from build123d import *

# Parameters (mm, degrees)
F0_R     = 114.3
F1_DEPTH = 15.24
F3_D     = 76.2
F5_D     = 20.32
F7_D     = 20.32


with BuildPart() as f1:
    # F0 (on Front) → F1 (new body)
    with BuildSketch(Plane.XZ):
        Circle(F0_R)
    extrude(amount=F1_DEPTH)

    # F3 (through all)
    with Locations(Plane.XZ.offset(15.24)):
        with Locations((0, 0)):
            Hole(F3_D / 2)

    # F5 (through all)
    with Locations(Plane.XZ.offset(15.24)):
        with Locations((0, 76.2)):
            Hole(F5_D / 2)

    # F7 (through all)
    with Locations(Plane.XZ.offset(15.24)):
        with Locations((0, -76.2)):
            Hole(F7_D / 2)


solid = f1.part
Could you check a few things on this model? Use its own coordinates, in mm. Give positions to 0.01 mm unless a question says otherwise; leave off trailing zeros. Order: outer loops, then holes, each group sorted by start corner. A loop starts at its lowest first (then second) coordinate and runs counter-clockwise, first axis right, second up. Notation, with made-up numbers: (57, 27) - (63, 27) arc R18 cw to (63, 31) - close; hole circle Ø4 at (-28.5, 88.5). An arc over 180 degrees is marked (long way). One line per question, with ' | ' between items. Start each with the question number.
Item 1: Thinking about a two-plate mould opening in Z: for faces 1 (the flat face through (-2, 0, -49)), 2 (the cylindrical face through (30.235, -7.513, -23.183)), 3 (the cylindrical face through (-114.19, -7.51, 5.03)), which applies, pulls with the +Z half, pulls with the -Z half, needs draft (parallel to the pull), parting line crosses it, or undercut?
Item 2: I want a section at D-D on y = -7.25. Write out the boundary of the cut face in (x, z).
Item 3: I'm going to push flat-ended pins straight in: pin 1 Ø4 at (y, z) = (-11, -58) entering from +X; pin 2 Ø6 at (y, z) = (-4, 15.5) entering from +X; pin 3 Ø1 at (x, y) = (38, -5) entering from +Z. Where does each tip first touch, or does it pass through?
Item 4: I need wall thicknesses on probe 1 along Z at (x, y) = (0, -3); probe 2 along X at (y, z) = (-0.75, -29); probe 3 along X at (y, z) = (-2.75, -18). Which ranges of each line are inside material? Lowest first, please. Write a range as [from, to].
Item 5: I want a section at B-B on z = 0. Write out the boundary of the cut face in (x, y).
Item 6: I want a section at A-A on x = 0. Write out the boundary of the cut face in (y, z).
Item 7: I want a section at C-C on x = 26. Write out the boundary of the cut face in (y, z).
Verdict:
1) face 1: needs draft | face 2: undercut | face 3: parting line crosses it
2) outline: circle Ø228.6 at (0, 0); hole circle Ø76.2 at (0, 0); hole circle Ø20.32 at (0, -76.2); hole circle Ø20.32 at (0, 76.2)
3) pin 1: x = 99.64 | pin 2: x = 113.61 | pin 3: z = 107.97
4) probe 1: [-114.3, -86.36], [-66.04, -38.1], [38.1, 66.04], [86.36, 114.3] | probe 2: [-110.56, -24.71], [24.71, 110.56] | probe 3: [-112.87, -33.58], [33.58, 112.87]
5) outline: (-114.3, -15.24) - (-38.1, -15.24) - (-38.1, 0) - (-114.3, 0) - close; (38.1, -15.24) - (114.3, -15.24) - (114.3, 0) - (38.1, 0) - close
6) outline: (-15.24, -114.3) - (0, -114.3) - (0, -86.36) - (-15.24, -86.36) - close; (-15.24, -66.04) - (0, -66.04) - (0, -38.1) - (-15.24, -38.1) - close; (-15.24, 38.1) - (0, 38.1) - (0, 66.04) - (-15.24, 66.04) - close; (-15.24, 86.36) - (0, 86.36) - (0, 114.3) - (-15.24, 114.3) - close
7) outline: (-15.24, -111.3) - (0, -111.3) - (0, -27.85) - (-15.24, -27.85) - close; (-15.24, 27.85) - (0, 27.85) - (0, 111.3) - (-15.24, 111.3) - close
